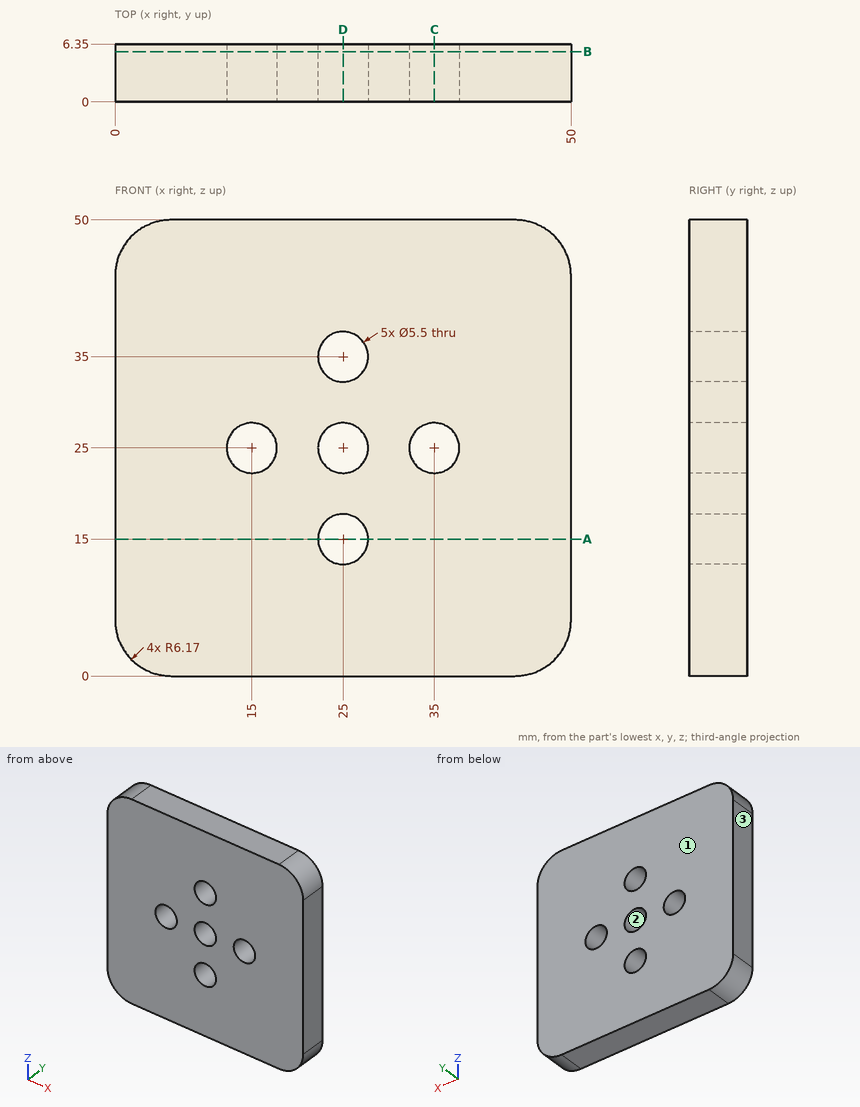
Answer from the drawing. Dimensions are ordinates in mm from the lowest x, y and z of the part. Give positions to 0.01 mm unless a question says otherwise; leave off trailing zeros. Order: outer loops, then holes, each group sorted by start corner. A loop starts at its lowest first (then second) coordinate and runs counter-clockwise, first axis right, second up. Notation, with made-up numbers: (59.5, -12) - (106.5, -12) arc R33 ccw to (106.5, 19) - close; hole circle Ø6 at (0, 13). An arc over 180 degrees is marked (long way). Use one line per item in the form item = value.
1) Consider probe 1 along Z at (x, y) = (25, 3.5); probe 2 along X at (y, z) = (4.5, 15). Determine where each line is inside the solid, lowest interval first. Write a range as [from, to].
Verdict:
probe_1 = [0, 12.25], [17.75, 22.25], [27.75, 32.25], [37.75, 50]
probe_2 = [0, 22.25], [27.75, 50]
2) The mould has two halves that part along X. Classify the marked faces 1, 2 and 3: released by +X, released by -X, zero draft, split by the parting line, or undercut.
Verdict:
face_1 = zero draft
face_2 = undercut
face_3 = released by -X
3) Find section C-C on x = 35. Determine the outline of the cut face in (y, z).
Verdict:
outline = (0, 0) - (6.35, 0) - (6.35, 22.25) - (0, 22.25) - close; (0, 27.75) - (6.35, 27.75) - (6.35, 50) - (0, 50) - close
4) Find section B-B on y = 5.5. Determine the outline of the cut face in (x, z).
Verdict:
outline = (0, 6.17) arc R6.17 ccw to (6.17, 0) - (43.83, 0) arc R6.17 ccw to (50, 6.17) - (50, 43.83) arc R6.17 ccw to (43.83, 50) - (6.17, 50) arc R6.17 ccw to (0, 43.83) - close; hole circle Ø5.5 at (15, 25); hole circle Ø5.5 at (25, 15); hole circle Ø5.5 at (25, 25); hole circle Ø5.5 at (25, 35); hole circle Ø5.5 at (35, 25)
5) This flat-tipped pin is pushed along its axis until it touches: pin 1 (7 mm diameter, centred on x = 25, z = 15, fed in from +Y). Where does it stop, or does it pass through?
Verdict:
pin_1 = 6.35
6) Find section D-D on x = 25. Determine the outline of the cut face in (y, z).
Verdict:
outline = (0, 0) - (6.35, 0) - (6.35, 12.25) - (0, 12.25) - close; (0, 17.75) - (6.35, 17.75) - (6.35, 22.25) - (0, 22.25) - close; (0, 27.75) - (6.35, 27.75) - (6.35, 32.25) - (0, 32.25) - close; (0, 37.75) - (6.35, 37.75) - (6.35, 50) - (0, 50) - close
7) Find section A-A on z = 15. Determine the outline of the cut face in (x, y), and give its area (3 significant figures).
Verdict:
outline = (0, 0) - (22.25, 0) - (22.25, 6.35) - (0, 6.35) - close; (27.75, 0) - (50, 0) - (50, 6.35) - (27.75, 6.35) - close
area = 283 mm^2
